Could you check a few things on this model? Use its own coordinates, in mm. A direction names the side the tool comes from. Give positions to 0.01 mm unless a question says otherwise; leave off trailing zeros. Loops run counter-clockwise (first coordinate to the right, second up) from the corner with the lowest first, then second, coordinate; pieces in that order, holes last. Notation, with made-up numbers: (41, 17.25) - (45, 17.25) arc R21 cw to (45, 54.25) - close; hole circle Ø7 at (82.5, 65.5). An arc over 180 degrees is marked (long way). Write each question's results on one line, items separated by ' | '. Start each with the question number.
Autodesk Inventor part; units mm, degrees
ref_plane "YZ Plane" through (0, 0, 0) normal (1, 0, 0) x (0, 1, 0)
ref_plane "XZ Plane" through (0, 0, 0) normal (0, 1, 0) x (-1, 0, 0)
ref_plane "XY Plane" through (0, 0, 0) normal (0, 0, 1) x (1, 0, 0)
sketch "Sketch1" plane through (0, 0, 0) normal (0, 1, 0) x (-1, 0, 0)
  line L0 (50.8, -50.8) -> (-50.8, -50.8)
  line L1 (50.8, -50.8) -> (50.8, 0)
  line L2 (-50.8, -50.8) -> (-50.8, 0)
  arc A0 (50.8, 0) -> (-50.8, 0) centre (0, 0) ccw
  line L3 (44.45, -44.45) -> (-44.45, -44.45)
  line L4 (-44.45, -44.45) -> (-44.45, 0)
  line L5 (44.45, -44.45) -> (44.45, 0)
  arc A1 (44.45, 0) -> (-44.45, 0) centre (0, 0) ccw
  dimension "d2" = 101.6
  dimension "d4" = 6.35
  dimension "d5" = 6.35
  dimension "d6" = 6.35
  dimension "d34" = 44.45
  dimension "d36" = 44.45
extrude "Extrusion1" add sketch "Sketch1" along normal blind 6.35
sketch "Sketch2" plane through (50.8, 0, -50.8) normal (0, 0, -1) x (-1, 0, 0)
  line L0 (101.6, 0) -> (101.6, 6.35)
  line L1 (0, 6.35) -> (101.6, 6.35)
  line L2 (0, 0) -> (0, 6.35)
  point P0 (50.8, 0)
  point P1 (3.175, 3.175)
  point P2 (98.425, 3.175)
  dimension "d9" = 3.175
  dimension "d10" = 3.175
  dimension "d11" = 3.175
hole "Hole1" at (47.625, 3.175, -50.8) at (-47.625, 3.175, -50.8) direction (0, 0, 1) diameter 4.826 depth 25.4
pattern_linear "Rectangular Pattern1" count 2 spacing 50.8 along (0, 1, 0) of "Extrusion1"
sketch "Sketch3" plane through (50.8, 50.8, -50.8) normal (0, 0, -1) x (-1, 0, 0)
  line L0 (101.6, 0) -> (101.6, 6.35)
  line L1 (0, 6.35) -> (101.6, 6.35)
  line L2 (0, 0) -> (0, 6.35)
  point P0 (50.8, -50.8)
  point P1 (3.175, 3.175)
  point P2 (98.425, 3.175)
  dimension "d22" = 3.175
  dimension "d23" = 3.175
  dimension "d24" = 3.175
hole "Hole2" at (47.625, 53.975, -50.8) at (-47.625, 53.975, -50.8) direction (0, 0, 1) diameter 4.826 depth 25.4
sketch "Sketch4" plane through (50.8, 50.8, -50.8) normal (0, 0, -1) x (-1, 0, 0)
  circle A0 centre (3.175, 3.175) radius 2.413
  circle A1 centre (98.425, 3.175) radius 2.413
  line L0 (101.6, 0) -> (0, 0) construction
  line L1 (0, 6.35) -> (101.6, 6.35)
  line L2 (0, 6.35) -> (101.6, 6.35)
  line L3 (0, 6.35) -> (101.6, 6.35)
  line L4 (101.6, 6.35) -> (101.6, -50.8)
  line L5 (101.6, -50.8) -> (0, -50.8)
  line L6 (0, -50.8) -> (0, 6.35)
  point P0 (50.8, -50.8)
extrude "Extrusion3" add sketch "Sketch4" along normal blind 5.08
equation "\"d5\" = d4"
equation "\"d6\" = d4"
properties part number "router_mount"
Q1. If we mould it in two halves opening along Z, with no side actions, what happens to faces 6 (the face through (0.98, 53.93, 44.44)), 7 (the face through (4, 50.8, -45)), 8 (the face through (1.117, 3.131, 50.788))? For each: +Z half, -Z half, draft (parallel to the pull), parting line (faces both ways), or undercut.
Q2. I want a section at B-B, the plane z = 3.5. List the corners of the cut face in (x, y) for me.
Q3. Which directions (+Z, -Z, +X, -X, +Y, -Y) give clear straight access to the entire face, cutting with the end or side of a thin tool? Please do faces 1 (the face through (48, 3, -50.8)), 2 (the face through (48, 54, -25.4)), 3 (the face through (4, 6.35, -45)), 4 (the face through (44.45, 3, -23)), 5 (the face through (4, 57.15, -46)).
Q4. I need wall thicknesses on L1, parallel to X at y = 52, z = -24; L2, parallel to Z at x = -28, y = 36; L3, parallel to Y at x = -44.5, z = -41.5. Which ranges of each line are inside material? Lowest first, please. Write a range as from..to.
Q5. I want a section at D-D, the plane z = 26.5. List the corners of the cut face in (x, y) for me.
Q6. I want a section at C-C, the plane x = -20. List the corners of the cut face in (y, z) for me, then the cut area to 3 significant figures.
Q7. I'm going to push flat-ended pins straight in: pin 1 Ø3 at (x, y) = (-47.625, 53.975) entering from -Z; pin 2 Ø3 at (x, y) = (-14, 10.5) entering from +Z; pin 3 Ø5.5 at (x, y) = (47.5, 4) entering from +Z; pin 4 Ø4 at (x, y) = (-46.5, 54) entering from -Z. Where does each tip first touch, or does it pass through?
Q8. I want a section at A-A, the plane x = 0. List the corners of the cut face in (y, z) for me.
Conclusion:
1) face 6: undercut | face 7: draft | face 8: +Z half
2) outline: (-50.68, 0) - (-44.31, 0) - (-44.31, 6.35) - (-50.68, 6.35) - close; (-50.68, 50.8) - (-44.31, 50.8) - (-44.31, 57.15) - (-50.68, 57.15) - close; (44.31, 0) - (50.68, 0) - (50.68, 6.35) - (44.31, 6.35) - close; (44.31, 50.8) - (50.68, 50.8) - (50.68, 57.15) - (44.31, 57.15) - close
3) face 1: none | face 2: -Z | face 3: +Z, +X, -X | face 4: +Y, -Y | face 5: +Z, -Z, +X, -X, +Y
4) L1: -50.8..-44.45, 44.45..50.8 | L2: -55.88..-50.8 | L3: 0..6.35, 50.8..57.15
5) outline: (-43.34, 0) - (-35.69, 0) - (-35.69, 6.35) - (-43.34, 6.35) - close; (-43.34, 50.8) - (-35.69, 50.8) - (-35.69, 57.15) - (-43.34, 57.15) - close; (35.69, 0) - (43.34, 0) - (43.34, 6.35) - (35.69, 6.35) - close; (35.69, 50.8) - (43.34, 50.8) - (43.34, 57.15) - (35.69, 57.15) - close
6) outline: (0, -55.88) - (57.15, -55.88) - (57.15, -44.45) - (50.8, -44.45) - (50.8, -50.8) - (6.35, -50.8) - (6.35, -44.45) - (0, -44.45) - close; (0, 39.7) - (6.35, 39.7) - (6.35, 46.7) - (0, 46.7) - close; (50.8, 39.7) - (57.15, 39.7) - (57.15, 46.7) - (50.8, 46.7) - close | area: 460 mm^2
7) pin 1: z = -25.4 | pin 2: z = -50.8 | pin 3: z = 24.04 | pin 4: z = -55.88
8) outline: (0, -55.88) - (57.15, -55.88) - (57.15, -44.45) - (50.8, -44.45) - (50.8, -50.8) - (6.35, -50.8) - (6.35, -44.45) - (0, -44.45) - close; (0, 44.45) - (6.35, 44.45) - (6.35, 50.8) - (0, 50.8) - close; (50.8, 44.45) - (57.15, 44.45) - (57.15, 50.8) - (50.8, 50.8) - close
